Geometry: see drawing. Coordinates: mm, zero at the bounding-box minimum. A direction names the side the tool comes from. Round coordinates to 2 decimals unless told otherwise and drop trailing zeros. Loops run counter-clockwise (first coordinate to the right, second up) from the corner with the lowest first, then second, coordinate; pieces in that order, holes last. Notation, with made-up numbers: (80, 25) -> (115, 25) arc R27 cw to (115, 61) -> close; hole circle Ø11 at (8.5, 33.5). An arc over 180 degrees is marked (long way). Answer in a Markdown table with one row per item.
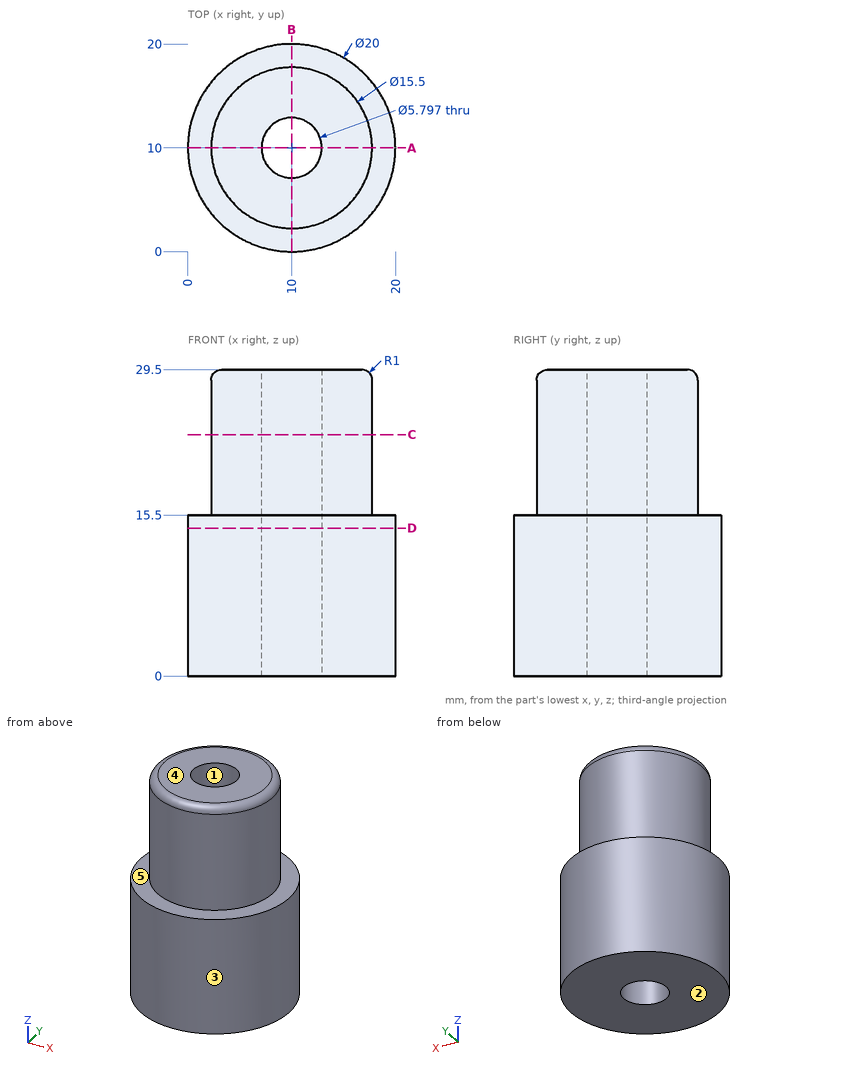
Item 1: Ray query, L1, parallel to Y at x = 10, z = 21.75; L2, parallel to Y at x = 10, z = 12.5; L3, parallel to Z at x = 11, y = 18. Return the intervals inside material, ascending.
Ans:
| item | result |
|---|---|
| L1 | 2.25 to 7.1, 12.9 to 17.75 |
| L2 | 0 to 7.1, 12.9 to 20 |
| L3 | 0 to 15.5 |
Item 2: Section query C-C, the plane z = 23.25. Output: boundary loops of the cut face in (x, y).
Ans:
| item | result |
|---|---|
| outline | circle Ø15.5 at (10, 10); hole circle Ø5.8 at (10, 10) |
Item 3: Set-up query: the marked faces 4 and 5. Return all of +Z, -Z, +X, -X, +Y, -Y with unobstructed straight access to the full face (end or side cutting, diameter ignored); none if empty.
Ans:
| item | result |
|---|---|
| face 4 | +Z, +X, -X, +Y, -Y |
| face 5 | +Z |
Item 4: Section query D-D, the plane z = 14.25. Output: boundary loops of the cut face in (x, y).
Ans:
| item | result |
|---|---|
| outline | circle Ø20 at (10, 10); hole circle Ø5.8 at (10, 10) |
Item 5: Mould query, pull axis X, two halves, no side actions, for the marked faces 1, 2 and 3. Classes: released by +X, released by -X, zero draft, split by the parting line, or undercut.
Ans:
| item | result |
|---|---|
| face 1 | undercut |
| face 2 | zero draft |
| face 3 | split by the parting line |
Item 6: First-contact query: P1, Ø3, axis at x = 12, z = 26.5, coming from the -Y side; P2, Ø10, axis at x = 4.5, z = 17, coming from the +Y side; P3, Ø8, axis at y = 14.5, z = 21.5, coming from the +X side. Flat tips, straight axial feed; report the tip coordinate or a pass-through.
Ans:
| item | result |
|---|---|
| P1 | y = 2.27 |
| P2 | y = 19.97 |
| P3 | x = 17.73 |
Item 7: Section query A-A, the plane y = 10. Output: boundary loops of the cut face in (x, z).
Ans:
| item | result |
|---|---|
| outline | (0, 0) -> (7.1, 0) -> (7.1, 29.5) -> (3.25, 29.5) arc R1 ccw to (2.25, 28.5) -> (2.25, 15.5) -> (0, 15.5) -> close; (12.9, 0) -> (20, 0) -> (20, 15.5) -> (17.75, 15.5) -> (17.75, 28.5) arc R1 ccw to (16.75, 29.5) -> (12.9, 29.5) -> close |
